from build123d import *

# Parameters (mm, degrees)
BOSS_EXTRUDE1_DEPTH = 104.775
BOSS_EXTRUDE2_DEPTH = 92.5957
BOSS_EXTRUDE3_START = -5.8293
BOSS_EXTRUDE3_DEPTH = 5.8293
BOSS_EXTRUDE4_DEPTH = 6.35
SKETCH5_W           = 7.787485422
SKETCH5_H           = 19.833751934
SKETCH5_W_2         = 22.754058967
SKETCH5_H_2         = 3.407024872
CUT_EXTRUDE1_DEPTH  = 227.312030137
SKETCH9_W           = 103.741840618
SKETCH9_H           = 106.576317138
CUT_EXTRUDE4_DEPTH  = 104.775
SKETCH10_W          = 104.775
SKETCH10_H          = 6.354337814
BOSS_EXTRUDE6_DEPTH = 6.35
FILLET2_R           = 6.35


with BuildPart() as part:
    # Sketch1 → Boss-Extrude1 (new, symmetric)
    with BuildSketch(Plane.XY):
        with BuildLine():
            Line((-58.2422, 56.2102), (-58.2422, 62.5602))
            ThreePointArc((-58.2422, 62.5602), (-45.640852469, 57.743322347), (-39.3748699, 45.7962))
            ThreePointArc((-39.3748699, 45.7962), (-25.556268964, 20.239931036), (0, 6.4213301))
            ThreePointArc((0, 6.4213301), (12.247457496, 0.293755183), (17.272, -12.446))
            Line((17.272, -12.446), (10.922, -12.446))
            ThreePointArc((10.922, -12.446), (7.760938146, -4.204686933), (0, 0))
            ThreePointArc((0, 0), (-30.011530905, 15.784669095), (-45.7962, 45.7962))
            ThreePointArc((-45.7962, 45.7962), (-50.144819563, 53.243313205), (-58.2422, 56.2102))
        make_face()
    extrude(amount=BOSS_EXTRUDE1_DEPTH, both=True)


with BuildPart() as boss_extrude2_tool:
    # Sketch2 → Boss-Extrude2 (new, symmetric)
    with BuildSketch(Plane.XY):
        with BuildLine():
            Line((-58.2422, 56.2102), (-58.2422, 45.796198296))
            Line((-58.2422, 45.796198296), (-45.796199685, 45.796198296))
            ThreePointArc((-45.796199685, 45.796198296), (-50.144818899, 53.243312648), (-58.2422, 56.2102))
        make_face()
        with BuildLine():
            Line((0, 0), (0, -12.446))
            Line((0, -12.446), (10.922, -12.446))
            ThreePointArc((10.922, -12.446), (7.760938146, -4.204686933), (0, 0))
        make_face()
    extrude(amount=BOSS_EXTRUDE2_DEPTH, both=True)


with BuildPart() as part_1:
    add(part.part)


with BuildPart() as part_2:
    # Boss-Extrude2: joined with boss_extrude2_tool
    add(part_1.part.fuse(boss_extrude2_tool.part, tol=0.00001))

    # Sketch3 → Boss-Extrude3 (add)
    with BuildSketch(Plane(origin=(0, 0, -104.775), x_dir=(-1, 0, 0), z_dir=(0, 0, -1)).offset(BOSS_EXTRUDE3_START)):
        with BuildLine():
            Line((58.2422, 56.2102), (58.2422, 45.796198296))
            Line((58.2422, 45.796198296), (45.7962, 45.7962))
            ThreePointArc((45.7962, 45.7962), (50.144819563, 53.243313205), (58.2422, 56.2102))
        make_face()
        with BuildLine():
            Line((0, 0), (0, -12.446))
            Line((0, -12.446), (-10.922, -12.446))
            ThreePointArc((-10.922, -12.446), (-7.760938146, -4.204686933), (0, 0))
        make_face()
    extrude(amount=BOSS_EXTRUDE3_DEPTH)

    # Sketch4 → Boss-Extrude4 (add)
    with BuildSketch(Plane.XY.offset(104.775)):
        with BuildLine():
            Line((-58.2422, 56.2102), (-58.2422, 45.796198296))
            Line((-58.2422, 45.796198296), (-45.7962, 45.7962))
            ThreePointArc((-45.7962, 45.7962), (-50.144819563, 53.243313205), (-58.2422, 56.2102))
        make_face()
        with BuildLine():
            Line((0, 0), (0, -12.446))
            Line((0, -12.446), (10.922, -12.446))
            ThreePointArc((10.922, -12.446), (7.760938146, -4.204686933), (0, 0))
        make_face()
    extrude(amount=-BOSS_EXTRUDE4_DEPTH)

    # Sketch5 → Cut-Extrude1 (cut, through all)
    with BuildSketch(Plane.XY.offset(104.775)):
        with Locations((-61.627942711, 54.680509116)):
            Rectangle(SKETCH5_W, SKETCH5_H)
        with Locations((8.225058429, -13.641512436)):
            Rectangle(SKETCH5_W_2, SKETCH5_H_2)
    extrude(amount=-CUT_EXTRUDE1_DEPTH, mode=Mode.SUBTRACT)

    # Sketch9 → Cut-Extrude4 (cut)
    with BuildSketch(Plane(origin=(0, 0, -104.775), x_dir=(-1, 0, 0), z_dir=(0, 0, -1))):
        with Locations((16.552204841, 26.535028587)):
            Rectangle(SKETCH9_W, SKETCH9_H)
    extrude(amount=-CUT_EXTRUDE4_DEPTH, mode=Mode.SUBTRACT)

    # Sketch10 → Boss-Extrude6 (add)
    with BuildSketch(Plane.ZY.offset(57.7342)):
        with Locations((52.3875, 59.374341949)):
            Rectangle(SKETCH10_W, SKETCH10_H)
    extrude(amount=BOSS_EXTRUDE6_DEPTH)

    # Fillet2
    # the kernel refuses this fillet: 6.35 mm, written as the material it takes off along each edge
    with BuildSketch(Plane(origin=(17.260151367, -11.938, -25.849178653), x_dir=(-0.30497213299383213, 0.9523612749882223, 0), z_dir=(0, 0, 1))) as fillet2_piece_1:
        with BuildLine():
            CenterArc((8.625598356, 6.114282737), FILLET2_R, 162.243512631, 123.416753829)
            Line((2.57810426, 8.050855782), (0, 0))
            ThreePointArc((0, 0), (5.169835731, -0.710949564), (10.339671461, 0))
        make_face()
    extrude(amount=156.473357306, mode=Mode.SUBTRACT)
    with BuildSketch(Plane(origin=(-64.0842, 62.551510856, -15.875), x_dir=(1, 0, 0), z_dir=(0, 0, 1))) as fillet2_piece_2:
        with BuildLine():
            CenterArc((FILLET2_R, -FILLET2_R), FILLET2_R, 90, 90)
            Line((0, -FILLET2_R), (0, 0))
            Line((0, 0), (FILLET2_R, 0))
        make_face()
    extrude(amount=136.525, mode=Mode.SUBTRACT)


solid = part_2.part
The listing builds one solid part. Answer for the finished solid, in the listing's coordinates (mm). A direction names the side the tool comes from. Give positions to 0.01 mm unless a question says otherwise; leave off trailing zeros. Write each loop counter-clockwise with the first axis right and the second up, starting at its lowest first coordinate (ties: lowest second). Pieces come first, ordered by that corner, then holes.
Item 1: Section B-B, the plane x = -53.5 is taken. Write down the section's boundary in (y, z) (3 decimals), plus the area to 3 significant figures.
Item 2: Find the intervals of material crossed by line 1 along Z through (x, y) = (4.5, -2.5) (3 decimals); line 2 along X through (y, z) = (-6, 11); line 3 along Y through (x, z) = (-14, 17), in increasing order.
Item 3: Section D-D, the plane x = 4 is taken. Write down the section's boundary in (y, z) (3 decimals).
Item 4: Flat-ended cylindrical pins translate along their axes: P1, Ø7, axis at y = 49, z = 103, coming from the -X side; P2, Ø8, axis at y = 21.5, z = 44, coming from the -X side; P3, Ø1.5, axis at x = -0.5, z = 60.5, coming from the -Y side; P4, Ø7, axis at y = -6, z = 101, coming from the -X side. Find the tip coordinate at first contact, or state that the pin passes through.
Item 5: Which of the six approach directions +Z, -Z, +X, -X, +Y, -Y give full straight-line access (tool end or side, diameter ignored) to faces 4 (the flat face through (4, -7, 98.425)), 5 (the flat face through (-52, 45.796, 102)), 6 (the cylindrical face through (-25.847, 20.533, 53.121))?
Item 6: Section C-C, the plane y = 11 is taken. Write down the section's boundary in (x, z) (3 decimals).
Item 7: Determine the mould class of faces 1 (the cylindrical face through (7.554, -3.975, 95.551)), 2 (the flat face through (-27, 20, 0)), 3 (the flat face through (4, -11.938, 47)) for opening direction Z: released by +Z, released by -Z, zero draft, split by the parting line, or undercut.
Completed:
1. outline: (45.796, 0) - (61.943, 0) - (61.943, 104.775) - (45.796, 104.775) - (45.796, 98.425) - (55.265, 98.425) - (55.265, 92.596) - (45.796, 92.596) - close
1. area: 1,640 mm2
2. line 1: z = 0 to 92.596, 98.425 to 104.775
2. line 2: x = 0 to 15.14
2. line 3: y = 4.52 to 11.58
3. outline: (-11.938, 0) - (5.589, 0) - (5.589, 104.775) - (-11.938, 104.775) - (-11.938, 98.425) - (-1.273, 98.425) - (-1.273, 92.596) - (-11.938, 92.596) - close
4. P1: stops at x = -57.73
4. P2: stops at x = -37.81
4. P3: stops at y = -11.94
4. P4: stops at x = 0
5. face 4: -X, -Y
5. face 5: +Z, -Z, -X, -Y
5. face 6: +Z, -Z, +X, +Y
6. outline: (-24.578, 0) - (-12.903, 0) - (-12.903, 104.775) - (-24.578, 104.775) - close
7. face 1: undercut
7. face 2: released by -Z
7. face 3: zero draft
